```python
from build123d import *

# Parameters (mm, degrees)
CHAMFER1_SIZE = 25.4


with BuildPart() as part:
    # Sketch1 → Revolve1 (revolve)
    with BuildSketch(Plane(origin=(0, 0, 0), x_dir=(0, 0, -1), z_dir=(1, 0, 0)), mode=Mode.PRIVATE) as revolve1_sk:
        with BuildLine():
            Line((-381, 762), (381, 762))
            Line((381, 762), (381, 1016))
            Line((381, 1016), (254, 1016))
            ThreePointArc((254, 1016), (0, 866.453801319), (-254, 1016))
            Line((-254, 1016), (-381, 1016))
            Line((-381, 1016), (-381, 762))
        make_face()
    revolve(revolve1_sk.sketch.rotate(Axis((0, 0, 0), (0, 0, -1)), 90), axis=Axis((0, 0, 0), (0, 0, -1)))

    # Chamfer1
    chamfer1_edges = [part.edges().sort_by_distance(p)[0] for p in [
        (-1016, 0, -381),
        (-762, 0, -381),
        (-762, 0, 381),
        (-1016, 0, 381),
    ]]
    chamfer(chamfer1_edges, length=CHAMFER1_SIZE)


solid = part.part
```
The model under review builds one solid part; all positions refer to its coordinate system, in mm. Coordinates: 2 decimals unless noted, no trailing zeros. Order: outer loops, then holes, each group sorted by start corner. A loop starts at its lowest first (then second) coordinate and runs counter-clockwise, first axis right, second up. Notation, with made-up numbers: M 22.5,-22 L 68.5,-22 A23 cw 68.5,-5 Z; hole C 18.25,83.25 d7. An arc over 180 degrees is marked long. One line per question, with ' | ' between items.
(1) For probe 1 along Y at (x, z) = (430, -124.5); probe 2 along X at (y, z) = (297.5, 285); probe 3 along Z at (x, y) = (-201, -907), list the stretches that pass through material, from the lowest coordinate up. Write a range as from..to.
Geometry results:
probe 1: y = -784.35..-629.08, 629.08..784.35 | probe 2: x = -971.47..-701.53, 701.53..971.47 | probe 3: z = -381..-180.07, 180.07..381
(2) Add section D-D, the plane z = -67. Write out the cut boundary in (x, y), then the cut area to 3 significant figures.
Geometry results:
outline: C 0,0 d1748.57; hole C 0,0 d1524 | area: 577,000 mm²
(3) Add section A-A, the plane y = 0. Write out the cut boundary in (x, z).
Geometry results:
outline: M -1016,-355.6 L -990.6,-381 L -787.4,-381 L -762,-355.6 L -762,355.6 L -787.4,381 L -990.6,381 L -1016,355.6 L -1016,254 A290.48 cw -1016,-254 Z; M 762,-355.6 L 787.4,-381 L 990.6,-381 L 1016,-355.6 L 1016,-254 A290.48 cw 1016,254 L 1016,355.6 L 990.6,381 L 787.4,381 L 762,355.6 Z
(4) Add section C-C, the plane z = -320.5. Write out the cut boundary in (x, y).
Geometry results:
outline: C 0,0 d2032; hole C 0,0 d1524
(5) Insertion check: pin 1 (1.5 mm diameter, centred on y = 431.5, z = -252, fed in from +X); pin 2 (1 mm diameter, centred on x = -663, z = -222, fed in from -Y); pin 3 (3 mm diameter, centred on x = -497, z = -277, fed in from -Y). Each pin has a flat end and moves straight along its axis. Give the tip position at first contact, or say it passes through.
Geometry results:
pin 1: stops at x = 917.4 | pin 2: stops at y = -708.44 | pin 3: stops at y = -886.98
(6) The part is to be moulded in two halves that separate along X. For faces 1 (the face through (-215.01, 968.248, 379.767)), 2 (the face through (-165.19, 743.88, -4.98)), 3 (the face through (665, 436, -381)), say which applies: +X half, -X half, draft (parallel to the pull), parting line (faces both ways), or undercut.
Geometry results:
face 1: parting line | face 2: undercut | face 3: draft
